from build123d import *

# Parameters (mm, degrees)
BOSS_EXTRUDE1_DEPTH              = 38.1
SKETCH2_W                        = 22.225
SKETCH2_H                        = 10.16
CUT_EXTRUDE1_DEPTH               = 3.175
SKETCH6_R                        = 1.5875
CUT_EXTRUDE2_DEPTH               = 3.175
SKETCH7_R                        = 4.7625
CUT_EXTRUDE3_DEPTH               = 3.175
F_1_4_0_25_DIAMETER_HOLE1_REACH  = 73.631
F_1_4_0_25_DIAMETER_HOLE1_BORE_R = 3.175


with BuildPart() as part:
    # Sketch1 → Boss-Extrude1 (new body)
    with BuildSketch(Plane(origin=(0, 0, 0), x_dir=(0, 0, -1), z_dir=(1, 0, 0))):
        Polygon((0, 0), (-38.1, 0), (-38.1, 41.275), (-41.275, 41.275), (-41.275, -3.175), (3.175, -3.175), (3.175, 22.225), (-22.225, 22.225), (-22.225, 19.05), (0, 19.05), align=None)
    extrude(amount=BOSS_EXTRUDE1_DEPTH)

    # Sketch2 → Cut-Extrude1 (cut)
    with BuildSketch(Plane(origin=(0, 22.225, 0), x_dir=(1, 0, 0), z_dir=(0, 1, 0))):
        with Locations((19.05, -17.145)):
            Rectangle(SKETCH2_W, SKETCH2_H)
    extrude(amount=-CUT_EXTRUDE1_DEPTH, mode=Mode.SUBTRACT)

    # Sketch6 → Cut-Extrude2 (cut)
    with BuildSketch(Plane(origin=(0, 22.225, 0), x_dir=(1, 0, 0), z_dir=(0, 1, 0))):
        with Locations(Location((33.3375, -3.175, 0), (0, 0, 270))):
            Circle(SKETCH6_R)
        with Locations(Location((4.7625, -3.175, 0), (0, 0, 270))):
            Circle(SKETCH6_R)
    extrude(amount=-CUT_EXTRUDE2_DEPTH, mode=Mode.SUBTRACT)

    # Sketch7 → Cut-Extrude3 (cut)
    with BuildSketch(Plane.XY.offset(41.275)):
        with Locations((19.05, 31.75)):
            Circle(SKETCH7_R)
    extrude(amount=-CUT_EXTRUDE3_DEPTH, mode=Mode.SUBTRACT)

    # 1/4 (0.25) Diameter Hole1 bore → 1/4 (0.25) Diameter Hole1 (cut, up to next)
    with BuildSketch(Plane(origin=(0, -3.175, 0), x_dir=(-1, 0, 0), z_dir=(0, -1, 0)), mode=Mode.PRIVATE) as f_1_4_0_25_diameter_hole1_sk1:
        with Locations((-19.05, -28.575)):
            Circle(F_1_4_0_25_DIAMETER_HOLE1_BORE_R)
    f_1_4_0_25_diameter_hole1_tool1 = extrude(f_1_4_0_25_diameter_hole1_sk1.sketch, amount=-F_1_4_0_25_DIAMETER_HOLE1_REACH, mode=Mode.PRIVATE) & part.part
    # 1/4 (0.25) Diameter Hole1 bore → 1/4 (0.25) Diameter Hole1 (cut, up to next)
    with BuildSketch(Plane(origin=(0, -3.175, 0), x_dir=(-1, 0, 0), z_dir=(0, -1, 0)), mode=Mode.PRIVATE) as f_1_4_0_25_diameter_hole1_sk2:
        with Locations((-19.05, -9.525)):
            Circle(F_1_4_0_25_DIAMETER_HOLE1_BORE_R)
    f_1_4_0_25_diameter_hole1_tool2 = extrude(f_1_4_0_25_diameter_hole1_sk2.sketch, amount=-F_1_4_0_25_DIAMETER_HOLE1_REACH, mode=Mode.PRIVATE) & part.part
    add(f_1_4_0_25_diameter_hole1_tool1.solids().sort_by_distance((19.05, -3.175, 28.575))[0], mode=Mode.SUBTRACT)
    add(f_1_4_0_25_diameter_hole1_tool2.solids().sort_by_distance((19.05, -3.175, 9.525))[0], mode=Mode.SUBTRACT)


solid = part.part
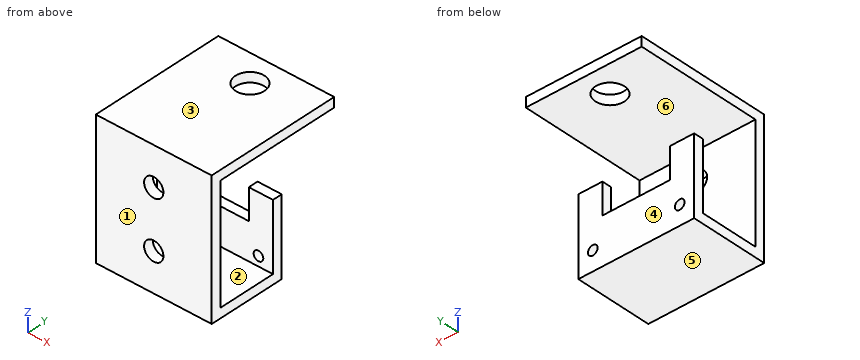
Input: part model. Units: mm. Frame: model coordinates. Face numbers are marked on the shaded views. A direction names the side the tool comes from. Round coordinates to 2 decimals unless told otherwise and drop trailing zeros. Order: outer loops, then holes, each group sorted by start corner. A loop starts at its lowest first (then second) coordinate and runs counter-clockwise, first axis right, second up.
1. Cut plane D-D, the plane z = 31. Output: boundary loops of the cut face in (x, y) (3 decimals).
The answers:
outline: (0, -3.175) - (17.001, -3.175) - (17.001, 0) - (0, 0) - close; (21.099, -3.175) - (38.1, -3.175) - (38.1, 0) - (21.099, 0) - close
2. Set-up query: the marked faces 1 and 2. Return all of +Z, -Z, +X, -X, +Y, -Y with unobstructed straight access to the full face (end or side cutting, diameter ignored); none if empty.
The answers:
face 1: +Z, -Z, +X, -X, -Y
face 2: +X, -X
3. Mould query, pull axis Z, two halves, no side actions, for the marked faces 3, 4, 5 and 6. Classes: released by +Z, released by -Z, zero draft, split by the parting line, or undercut.
The answers:
face 3: released by +Z
face 4: zero draft
face 5: released by -Z
face 6: undercut
4. Pin query (flat end, axial travel): P1, Ø3, axis at x = 22.5, y = 30.5, coming from the -Z side; P2, Ø8, axis at x = 26, z = 9, coming from the +Y side (3 decimals); P3, Ø1.6, axis at y = 21, z = 16, coming from the -X side; P4, Ø3, axis at x = 25, z = 31.5, coming from the +Y side. Return the tip coordinate at first contact, or that it passes through.
The answers:
P1: stops at z = 38.1
P2: stops at y = 22.225
P3: stops at x = 0
P4: stops at y = 0
5. Cut plane A-A, the plane z = 20. State how many separate pieces and enclosed holes the cut face has, then the cut area to 3 significant figures.
The answers:
separate pieces: 3
enclosed holes: 0
area: 171 mm2
6. Cut plane C-C, the plane y = 31.75. Output: boundary loops of the cut face in (x, z) (1 decimal).
The answers:
outline: (0, 38.1) - (14.3, 38.1) - (14.3, 41.3) - (0, 41.3) - close; (23.8, 38.1) - (38.1, 38.1) - (38.1, 41.3) - (23.8, 41.3) - close
7. Material intervals for line 1 (Z direction, x = 19.05, y = -0.8) (3 decimals); line 2 (Z direction, x = 28.5, y = 18) (3 decimals); line 3 (Y direction, x = 28.5, z = 1) (3 decimals), sorted ascending.
The answers:
line 1: z = -3.175 to 6.35, 12.7 to 25.4, 31.75 to 41.275
line 2: z = -3.175 to 0, 38.1 to 41.275
line 3: y = -3.175 to 0, 19.05 to 22.225
